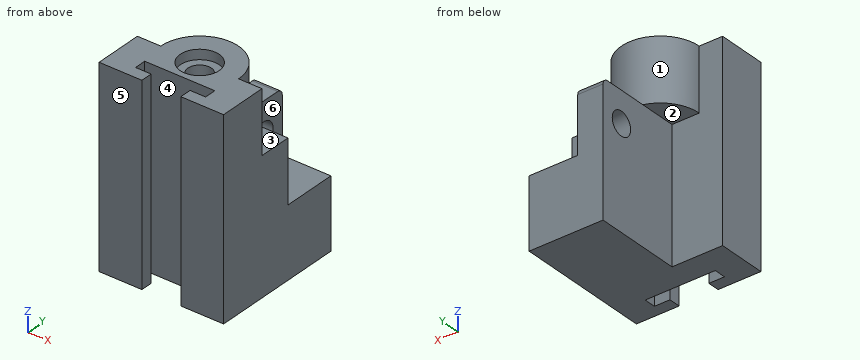
```python
from build123d import *

# Parameters (mm, degrees)
SKETCH1_W                                    = 64
SKETCH1_H                                    = 100
BOSS_EXTRUDE1_DEPTH                          = 25
SKETCH2_W                                    = 38
SKETCH2_H                                    = 68
BOSS_EXTRUDE2_DEPTH                          = 45
SKETCH3_W                                    = 32
SKETCH3_H                                    = 28
CUT_EXTRUDE1_DEPTH                           = 25
BOSS_EXTRUDE3_DEPTH                          = 32
CUT_EXTRUDE2_DEPTH                           = 127.968500031
FILLET1_R                                    = 3
CBORE_FOR_M10_CHEESE_HEAD_SCREW1_D           = 12
CBORE_FOR_M10_CHEESE_HEAD_SCREW1_DEPTH       = 25
CBORE_FOR_M10_CHEESE_HEAD_SCREW1_CBORE_D     = 20
CBORE_FOR_M10_CHEESE_HEAD_SCREW1_CBORE_DEPTH = 5
SKETCH7_R                                    = 6
CUT_EXTRUDE3_DEPTH                           = 117.387284529


with BuildPart() as part:
    # Sketch1 → Boss-Extrude1 (new body)
    with BuildSketch(Plane(origin=(0, 0, 0), x_dir=(1, 0, 0), z_dir=(0, 1, 0))):
        with Locations((32, 50)):
            Rectangle(SKETCH1_W, SKETCH1_H)
    extrude(amount=-BOSS_EXTRUDE1_DEPTH)

    # Sketch2 → Boss-Extrude2 (add)
    with BuildSketch(Plane(origin=(0, 0, 0), x_dir=(1, 0, 0), z_dir=(0, 1, 0))):
        with Locations((45, 66)):
            Rectangle(SKETCH2_W, SKETCH2_H)
    extrude(amount=BOSS_EXTRUDE2_DEPTH)

    # Sketch3 → Cut-Extrude1 (cut)
    with BuildSketch(Plane(origin=(64, 0, 0), x_dir=(0, 0, -1), z_dir=(1, 0, 0))):
        with Locations((48, 31)):
            Rectangle(SKETCH3_W, SKETCH3_H)
    extrude(amount=-CUT_EXTRUDE1_DEPTH, mode=Mode.SUBTRACT)

    # Sketch4 → Boss-Extrude3 (add)
    with BuildSketch(Plane.XY):
        with BuildLine():
            ThreePointArc((52, 0), (32, 20), (12, 0))
            Line((12, 0), (52, 0))
        make_face()
    extrude(amount=-BOSS_EXTRUDE3_DEPTH)

    # Sketch4<3> → Cut-Extrude2 (cut, through all)
    with BuildSketch(Plane.XY):
        Polygon((22, -19), (22, -25), (42, -25), (42, -19), (50, -19), (50, -13), (14, -13), (14, -19), align=None)
    extrude(amount=-CUT_EXTRUDE2_DEPTH, mode=Mode.SUBTRACT)

    # Fillet1
    fillet1_edges = [part.edges().sort_by_distance(p)[0] for p in [
        (32.5, 45, -32),
    ]]
    fillet(fillet1_edges, radius=FILLET1_R)

    # CBORE for M10 Cheese Head Screw1
    with Locations(Plane.XY):
        with Locations((32, 0)):
            CounterBoreHole(CBORE_FOR_M10_CHEESE_HEAD_SCREW1_D / 2, CBORE_FOR_M10_CHEESE_HEAD_SCREW1_CBORE_D / 2, CBORE_FOR_M10_CHEESE_HEAD_SCREW1_CBORE_DEPTH, depth=CBORE_FOR_M10_CHEESE_HEAD_SCREW1_DEPTH)

    # Sketch7 → Cut-Extrude3 (cut, through all)
    with BuildSketch(Plane(origin=(39, 0, 0), x_dir=(0, 0, -1), z_dir=(1, 0, 0))):
        with Locations((48, 33)):
            Circle(SKETCH7_R)
    extrude(amount=-CUT_EXTRUDE3_DEPTH, mode=Mode.SUBTRACT)


solid = part.part
```
Read the model definition and answer for the solid it produces. Units are mm, in the model's axes. Face numbers are marked on the shaded views. A direction names the side the tool comes from. Give positions to 0.01 mm unless a question says otherwise; leave off trailing zeros. Order: outer loops, then holes, each group sorted by start corner. A loop starts at its lowest first (then second) coordinate and runs counter-clockwise, first axis right, second up.
(1) Find section B-B (y = 33). Give the vertices of the cut face in (x, z), plus the area to 3 significant figures.
(2) Find section A-A (z = -48). Give the vertices of the cut face in (x, y), plus the area to 3 significant figures.
(3) For a pull along Y with two mould halves and no side action, classify the marked faces 4, 5 and 6 as released by +Y, released by -Y, zero draft, split by the parting line, or undercut.
(4) Straight lines are drawn through the part: L1, parallel to Y at x = 35.75, z = -48; L2, parallel to Y at x = 32, z = -9; L3, parallel to Z at x = 60, y = 29. For each, find the intervals that lie inside material, in ascending order.
(5) Find section D-D (x = 15.5). Give the vertices of the cut face in (y, z).
(6) Find section C-C (z = -12). Give the vertices of the cut face in (x, y).
(7) For the marked faces 1, 2 and 3, determine the directions among +Z, -Z, +X, -X, +Y, -Y from which every point of the face is accessible in a straight line to the end or side of a thin tool.
(8) Given pin 1 (12 mm diameter, centred on x = 36.5, z = -28.5, fed in from +Y); pin 2 (9 mm diameter, centred on x = 20, z = -48, fed in from +Y); pin 3 (2 mm diameter, centred on y = 10.5, z = -54, fed in from -X), each flat-ended and moving along its own axis, determine where each tip first touches the part or whether it passes through.
Result sheet:
1. outline: (26, -100) - (64, -100) - (64, -64) - (39, -64) - (39, -54) - (26, -54) - close; (26, -42) - (39, -42) - (39, -32) - (26, -32) - close
1. area: 1,630 mm2
2. outline: (0, -25) - (22, -25) - (22, -19) - (14, -19) - (14, -13) - (50, -13) - (50, -19) - (42, -19) - (42, -25) - (64, -25) - (64, 17) - (39, 17) - (39, 27) - (26, 27) - (26, 0) - (0, 0) - close; (26, 39) - (39, 39) - (39, 45) - (26, 45) - close
2. area: 2,120 mm2
3. face 4: undercut
3. face 5: released by -Y
3. face 6: zero draft
4. L1: y = -13 to 27, 39 to 45
4. L2: y = -13 to -6, 6 to 20
4. L3: z = -100 to -64
5. outline: (-25, -100) - (-19, -100) - (-19, 0) - (-25, 0) - close; (-13, -100) - (0, -100) - (0, -32) - (11.3, -32) - (11.3, 0) - (-13, 0) - close
6. outline: (0, -25) - (22, -25) - (22, -19) - (14, -19) - (14, -13) - (50, -13) - (50, -19) - (42, -19) - (42, -25) - (64, -25) - (64, 0) - (52, 0) arc R20 ccw to (12, 0) - (0, 0) - close; hole circle Ø12 at (32, 0)
7. face 1: +Z, +Y
7. face 2: -Z, -X, +Y
7. face 3: +Z, +X, +Y
8. pin 1: stops at y = 44.96
8. pin 2: stops at y = 0
8. pin 3: stops at x = 26
